from build123d import *

# Parameters (mm, degrees)
BOSS_EXTRUDE1_DEPTH     = 10.8
CUT_EXTRUDE1_DEPTH      = 63.509359299
CUT_EXTRUDE1_DEPTH_BACK = 63.509359299
SKETCH14_W              = 32
SKETCH14_H              = 30
CUT_EXTRUDE3_DEPTH      = 60.51688836
FILLET1_R               = 3
SKETCH16_R              = 1.6
CUT_EXTRUDE2_DEPTH      = 60.51688836
CUT_EXTRUDE4_DEPTH      = 75.590213715
BOSS_EXTRUDE3_START     = -2.5
SKETCH22_R              = 1.65
BOSS_EXTRUDE3_DEPTH     = 2.5
BOSS_EXTRUDE4_START     = 7.1
SKETCH24_R              = 3.6
SKETCH24_R_2            = 1.6
BOSS_EXTRUDE4_DEPTH     = 7.1
CHAMFER1_SIZE           = 1


with BuildPart() as part:
    # Sketch6 → Revolve1 (revolve)
    with BuildSketch(Plane(origin=(0, 0, 0), x_dir=(0, 0, -1), z_dir=(1, 0, 0)), mode=Mode.PRIVATE) as revolve1_sk:
        Polygon((-2, 25.4), (-2, 35.1), (-25, 35.1), (-25, 37.95), (-12, 37.95), (-12, 41.1), (-9.5, 41.1), (-9.5, 38.1), (0, 38.1), (0, 25.4), (0, 0), (-2, 0), align=None)
    revolve(revolve1_sk.sketch.rotate(Axis((0, 0, 0), (0, 0, 1)), 90), axis=Axis((0, 0, 0), (0, 0, 1)))

    # Sketch15 → Boss-Extrude1 (add)
    with BuildSketch(Plane.XY.offset(2)):
        with BuildLine():
            Line((-20, 15.904297927), (20, 15.904297927))
            ThreePointArc((20, 15.904297927), (22.121320344, 15.02561827), (23, 12.904297927))
            Line((23, 12.904297927), (23, -24.995702073))
            ThreePointArc((23, -24.995702073), (22.121320344, -27.117022417), (20, -27.995702073))
            Line((20, -27.995702073), (-20, -27.995702073))
            ThreePointArc((-20, -27.995702073), (-22.121320344, -27.117022417), (-23, -24.995702073))
            Line((-23, -24.995702073), (-23, 12.904297927))
            ThreePointArc((-23, 12.904297927), (-22.121320344, 15.02561827), (-20, 15.904297927))
        make_face()
    extrude(amount=BOSS_EXTRUDE1_DEPTH)

    # Sketch14 → Cut-Extrude1 (cut, two sides: drawn at the far end of the back side and taken through both)
    with BuildSketch(Plane.XY.offset(2).offset(-CUT_EXTRUDE1_DEPTH_BACK)):
        with Locations((-0.00164643, -5.995702073)):
            Rectangle(SKETCH14_W, SKETCH14_H)
    extrude(amount=CUT_EXTRUDE1_DEPTH + CUT_EXTRUDE1_DEPTH_BACK, mode=Mode.SUBTRACT)

    # Sketch18 → Cut-Extrude3 (cut, through all)
    with BuildSketch(Plane.XY.offset(12.8)):
        with BuildLine():
            Line((19.99835357, -24.995702073), (23.99835357, -24.995702073))
            Line((23.99835357, -24.995702073), (23.99835357, -25.995702073))
            ThreePointArc((23.99835357, -25.995702073), (23.119673914, -28.117022417), (20.99835357, -28.995702073))
            Line((20.99835357, -28.995702073), (19.99835357, -28.995702073))
            Line((19.99835357, -28.995702073), (19.99835357, -24.995702073))
        make_face()
        with BuildLine():
            Line((-20.00164643, -24.995702073), (-24.00164643, -24.995702073))
            Line((-24.00164643, -24.995702073), (-24.00164643, -25.995702073))
            ThreePointArc((-24.00164643, -25.995702073), (-23.122966774, -28.117022417), (-21.00164643, -28.995702073))
            Line((-21.00164643, -28.995702073), (-20.00164643, -28.995702073))
            Line((-20.00164643, -28.995702073), (-20.00164643, -24.995702073))
        make_face()
    extrude(amount=CUT_EXTRUDE3_DEPTH, mode=Mode.SUBTRACT)

    # Fillet1
    fillet1_edges = [part.edges().sort_by_distance(p)[0] for p in [
        (-16.00164643, 9.004297927, 6.4),
        (-16.00164643, -20.995702073, 6.4),
        (15.99835357, -20.995702073, 6.4),
        (15.99835357, 9.004297927, 6.4),
    ]]
    fillet(fillet1_edges, radius=FILLET1_R)

    # Sketch16 → Cut-Extrude2 (cut, through all)
    with BuildSketch(Plane.XY.offset(12.8)):
        with Locations((-20.00164643, 13.004297927)):
            Circle(SKETCH16_R)
        with Locations((-20.00164643, -24.995702073)):
            Circle(SKETCH16_R)
        with Locations((19.99835357, -24.995702073)):
            Circle(SKETCH16_R)
        with Locations((19.99835357, 13.004297927)):
            Circle(SKETCH16_R)
    extrude(amount=-CUT_EXTRUDE2_DEPTH, mode=Mode.SUBTRACT)

    # Sketch20 → Cut-Extrude4 (cut, through all)
    with BuildSketch(Plane(origin=(0, 15.904297927, 0), x_dir=(1, 0, 0), z_dir=(0, 1, 0))):
        Polygon((20, -12.8), (-20, -12.8), (-20, -25), (19.99835357, -25), align=None)
    extrude(amount=CUT_EXTRUDE4_DEPTH, mode=Mode.SUBTRACT)

    # Sketch22 → Boss-Extrude3 (add)
    # profile 1 of 2: a face of its own
    with BuildSketch(Plane.XY.offset(12).offset(BOSS_EXTRUDE3_START)):
        with BuildLine():
            Line((-40.237833378, 34.580979128), (-31.752552003, 26.095697754))
            ThreePointArc((-31.752552003, 26.095697754), (-29.062088707, 29.062088707), (-26.095697754, 31.752552003))
            Line((-26.095697754, 31.752552003), (-34.580979128, 40.237833378))
            Line((-34.580979128, 40.237833378), (-40.237833378, 34.580979128))
        make_face()
        with Locations((-34.580979128, 34.580979128)):
            Circle(SKETCH22_R, mode=Mode.SUBTRACT)
    # profile 2 of 2: a face of its own
    with BuildSketch(Plane.XY.offset(12).offset(BOSS_EXTRUDE3_START)):
        with BuildLine():
            ThreePointArc((26.095697754, 31.752552003), (29.062088707, 29.062088707), (31.752552003, 26.095697754))
            Line((31.752552003, 26.095697754), (40.237833378, 34.580979128))
            Line((40.237833378, 34.580979128), (34.580979128, 40.237833378))
            Line((34.580979128, 40.237833378), (26.095697754, 31.752552003))
        make_face()
        with Locations((34.580979128, 34.580979128)):
            Circle(SKETCH22_R, mode=Mode.SUBTRACT)
    boss_extrude3 = extrude(amount=BOSS_EXTRUDE3_DEPTH)

    # Sketch24 → Boss-Extrude4 (add)
    # profile 1 of 4: a face of its own
    with BuildSketch(Plane.XY.offset(12.8).offset(BOSS_EXTRUDE4_START)):
        with Locations(Location((-20.00164643, 13.004297927, 0), (0, 0, 213.6046846))):
            Circle(SKETCH24_R)
        with Locations((-20.00164643, 13.004297927)):
            Circle(SKETCH24_R_2, mode=Mode.SUBTRACT)
    # profile 2 of 4: a face of its own
    with BuildSketch(Plane.XY.offset(12.8).offset(BOSS_EXTRUDE4_START)):
        with Locations(Location((19.99835357, 13.004297927, 0), (0, 0, 126.336057515))):
            Circle(SKETCH24_R)
        with Locations((19.99835357, 13.004297927)):
            Circle(SKETCH24_R_2, mode=Mode.SUBTRACT)
    # profile 3 of 4: a face of its own
    with BuildSketch(Plane.XY.offset(12.8).offset(BOSS_EXTRUDE4_START)):
        with Locations(Location((-20.00164643, -24.995702073, 0), (0, 0, 198.741091164))):
            Circle(SKETCH24_R)
        with Locations((-20.00164643, -24.995702073)):
            Circle(SKETCH24_R_2, mode=Mode.SUBTRACT)
    # profile 4 of 4: a face of its own
    with BuildSketch(Plane.XY.offset(12.8).offset(BOSS_EXTRUDE4_START)):
        with Locations(Location((19.99835357, -24.995702073, 0), (0, 0, 236.442690237))):
            Circle(SKETCH24_R)
        with Locations((19.99835357, -24.995702073)):
            Circle(SKETCH24_R_2, mode=Mode.SUBTRACT)
    extrude(amount=-BOSS_EXTRUDE4_DEPTH)

    # Chamfer1
    chamfer1_edges = [part.edges().sort_by_distance(p)[0] for p in [
        (-21.60164643, 13.004297927, 19.9),
        (18.39835357, 13.004297927, 19.9),
        (-21.60164643, -24.995702073, 19.9),
        (18.39835357, -24.995702073, 19.9),
    ]]
    chamfer(chamfer1_edges, length=CHAMFER1_SIZE)

    # Mirror1: Boss-Extrude3 across plane
    add(boss_extrude3.mirror(Plane.ZX))


solid = part.part
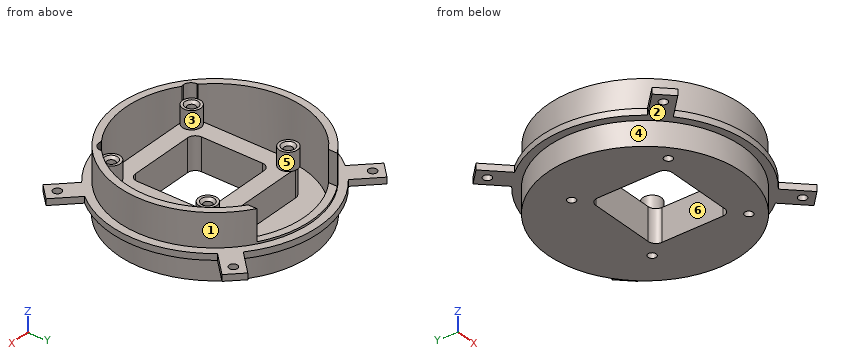
For this review, take the finished solid that the model builds, in its own axes (mm). Face numbers are marked on the shaded views. A direction names the side the tool comes from. Round coordinates to 2 decimals unless told otherwise and drop trailing zeros. Loops run counter-clockwise (first coordinate to the right, second up) from the corner with the lowest first, then second, coordinate; pieces in that order, holes last. Notation, with made-up numbers: (-36, -24.5) - (-11, -24.5) arc R7 cw to (-11, -19.5) - close; hole circle Ø1 at (-19, -40). An arc over 180 degrees is marked (long way). Put each result on its own line as item: value. Start each with the question number.
1. Consider section D-D on z = 14.5. State how many separate pieces and enclosed holes the cut face has, plus the area to 3 significant figures.
2. Mouldability with a two-part tool opening along X and no side actions: class the marked faces 1, 2 and 3 as +X half, -X half, draft (parallel to the pull), parting line (faces both ways), or undercut.
3. Insertion check: P1, Ø1, axis at x = 16.5, z = 12, coming from the -Y side; P2, Ø7.5, axis at x = -9.5, y = 32.5, coming from the +Z side; P3, Ø3, axis at x = 7, z = 9, coming from the -Y side; P4, Ø2, axis at x = 34.58, y = 34.58, coming from the +Z side. Each pin has a flat end and moves straight along its axis. Give the tip position at first contact, or say it passes through.
4. For probe 1 along Y at (x, z) = (-13, 9); probe 2 along X at (y, z) = (-2, 7.5); probe 3 along X at (y, z) = (-24, 2.75), list the stretches that pass through material, from the lowest coordinate up. Write a range as [from, to].
5. Consider section C-C on y = 0. State the section outline as (x, z) points.
6. Consider section B-B on x = 0. State the section outline as (y, z) points.
7. Consider section A-A on z = 4.5. State the section outline as (x, y) points.
8. For the marked faces 4, 5 and 6, list the 3-axis set-ups (+Z, -Z, +X, -X, +Y, -Y) from which the entire face can be reached by the end or side of a thin tool; tool diameter is ignored.
Result sheet:
1. separate pieces: 5
1. enclosed holes: 4
1. area: 654 mm^2
2. face 1: parting line
2. face 2: draft
2. face 3: undercut
3. P1: y = -37.86
3. P2: z = 12.8
3. P3: y = -40.72
3. P4: through
4. probe 1: [-35.81, -32.6], [-28, -21], [9, 15.9], [32.6, 35.81]
4. probe 2: [-38.05, -35.04], [-23, -16], [16, 23], [35.04, 38.05]
4. probe 3: [-29.59, -25.61], [-23, -21.25], [-18.75, 18.75], [21.25, 23], [25.61, 29.59]
5. outline: (-41.1, 9.5) - (-38.1, 9.5) - (-38.1, 0) - (-16, 0) - (-16, 12.8) - (-23, 12.8) - (-23, 2) - (-35.1, 2) - (-35.1, 25) - (-37.95, 25) - (-37.95, 12) - (-41.1, 12) - close; (16, 0) - (38.1, 0) - (38.1, 9.5) - (41.1, 9.5) - (41.1, 12) - (37.95, 12) - (37.95, 25) - (35.1, 25) - (35.1, 2) - (23, 2) - (23, 12.8) - (16, 12.8) - close
6. outline: (-41.1, 9.5) - (-38.1, 9.5) - (-38.1, 0) - (-21, 0) - (-21, 12.8) - (-28, 12.8) - (-28, 2) - (-35.1, 2) - (-35.1, 25) - (-37.95, 25) - (-37.95, 12) - (-41.1, 12) - close; (9, 0) - (38.1, 0) - (38.1, 9.5) - (41.1, 9.5) - (41.1, 12) - (37.95, 12) - (37.95, 12.8) - (35.1, 12.8) - (35.1, 2) - (15.9, 2) - (15.9, 12.8) - (9, 12.8) - close
7. outline: circle Ø76.2 at (0, 0); (-23, -25) arc R3 ccw to (-20, -28) - (20, -28) arc R3 ccw to (23, -25) - (23, 12.9) arc R3 ccw to (20, 15.9) - (-20, 15.9) arc R3 ccw to (-23, 12.9) - close; hole circle Ø70.2 at (0, 0); hole circle Ø3.2 at (-20, -25); hole circle Ø3.2 at (-20, 13); hole (-16, -18) arc R3 ccw to (-13, -21) - (13, -21) arc R3 ccw to (16, -18) - (16, 6) arc R3 ccw to (13, 9) - (-13, 9) arc R3 ccw to (-16, 6) - close; hole circle Ø3.2 at (20, -25); hole circle Ø3.2 at (20, 13)
8. face 4: -Z
8. face 5: +Z
8. face 6: +Z, -Z
